from build123d import *

# Parameters (mm, degrees)
SKETCH1_R               = 0.5
SKETCH1_R_2             = 3.4
SKETCH1_R_3             = 2.2
SKETCH1_R_4             = 1.25
BASE_DEPTH              = 2.08
SKETCH1_3_R             = 3.4
SKETCH1_3_R_2           = 2.2
CONNECTION_DEPTH        = 2.5
CONNECTION_DEPTH_BACK   = 2.25
SKETCH2_W               = 9.1
SKETCH2_H               = 3.75
ALIGNMENT_CHANNEL_DEPTH = 10


with BuildPart() as part:
    # Sketch1 → Base (new body)
    with BuildSketch(Plane.XY):
        with BuildLine():
            ThreePointArc((16.424, -1.942221409), (18.2, 0), (16.424, 1.942221409))
            Line((16.424, 1.942221409), (0.303384615, 3.386437328))
            ThreePointArc((0.303384615, 3.386437328), (2.509134083, 2.294394507), (3.4, 0))
            ThreePointArc((3.4, 0), (2.509134083, -2.294394507), (0.303384615, -3.386437328))
            Line((0.303384615, -3.386437328), (16.424, -1.942221409))
        make_face()
        with Locations((5.1, 0)):
            Circle(SKETCH1_R, mode=Mode.SUBTRACT)
        with Locations((6.983333333, 0)):
            Circle(SKETCH1_R, mode=Mode.SUBTRACT)
        with Locations((8.866666667, 0)):
            Circle(SKETCH1_R, mode=Mode.SUBTRACT)
        with Locations((10.75, 0)):
            Circle(SKETCH1_R, mode=Mode.SUBTRACT)
        with Locations((12.633333333, 0)):
            Circle(SKETCH1_R, mode=Mode.SUBTRACT)
        with Locations((14.516666667, 0)):
            Circle(SKETCH1_R, mode=Mode.SUBTRACT)
        with Locations((16.4, 0)):
            Circle(SKETCH1_R, mode=Mode.SUBTRACT)
        Circle(SKETCH1_R_2)
        Circle(SKETCH1_R_3, mode=Mode.SUBTRACT)
        Circle(SKETCH1_R_3)
        Circle(SKETCH1_R_4, mode=Mode.SUBTRACT)
    extrude(amount=BASE_DEPTH)

    # Sketch1_3 → Connection (add, two sides)
    with BuildSketch(Plane.XY) as connection_sk:
        Circle(SKETCH1_3_R)
        Circle(SKETCH1_3_R_2, mode=Mode.SUBTRACT)
    extrude(amount=CONNECTION_DEPTH)
    extrude(connection_sk.sketch, amount=-CONNECTION_DEPTH_BACK)

    # Sketch2 → Alignment channel (cut)
    with BuildSketch(Plane(origin=(0, 0, 0), x_dir=(-1, 0, 0), z_dir=(0, 0, -1))):
        with Locations((-8.575, 0)):
            Rectangle(SKETCH2_W, SKETCH2_H)
    extrude(amount=-ALIGNMENT_CHANNEL_DEPTH, mode=Mode.SUBTRACT)


solid = part.part
Verification items for the finished model (mm, model axes). A direction names the side the tool comes from. Give positions to 0.01 mm unless a question says otherwise; leave off trailing zeros. Loops run counter-clockwise (first coordinate to the right, second up) from the corner with the lowest first, then second, coordinate; pieces in that order, holes last. Notation, with made-up numbers: (-25.75, 69) - (-10.75, 69) arc R13 cw to (-10.75, 80) - close; hole circle Ø6 at (56, -36). An arc over 180 degrees is marked (long way). Write item = value, one per line. Start each with the question number.
Q1. Cross-section at D-D, the plane x = 5.5. Enter the section's corners in (y, z) (3 decimals), and give its area (3 significant figures).
Q2. Thickness scan on line 1 (Y direction, x = 0, z = 0.6); line 2 (Y direction, x = 0, z = -1.45); line 3 (X direction, y = -0.75, z = 1.15) (3 decimals). Record the ranges inside material, lowest first.
Q3. Cross-section at A-A, the plane x = 0. Enter the section's corners in (y, z).
Q4. Cross-section at C-C, the plane y = -1. Enter the section's corners in (x, z) (3 decimals).
Q5. Depth check by flat-ended pin: P1, Ø2, axis at x = 8, z = 0, coming from the -Y side; P2, Ø0.5, axis at y = 1, z = 1, coming from the -X side; P3, Ø2, axis at x = 1, y = 0.5, coming from the -Z side. Enter the tip coordinate at first touch or a pass-through.
Q6. Tool access check on faces 1 (the face through (2.1, 0.66, -1.11)), 2 (the face through (18.2, 0, 1)), 3 (the face through (4.025, 0, 1)), 4 (the face through (2.1, 0.66, 2.29)), 5 (the face through (-2, 2, 2.5)). Record the directions out of +Z, -Z, +X, -X, +Y, -Y that give a thin tool (end or side, any length) a straight path to the whole face; none if there is none.
Q7. Cross-section at B-B, the plane z = 1.8. Enter the section's corners in (x, y) (3 decimals), and give its area (3 significant figures).
Q8. Mould release check, pull along X, two halves, no side actions. Record for faces 6 (the face through (-3.4, 0.1, 0.2)), 7 (the face through (9, 1.875, 1)), 8 (the face through (-2, 2, -2.25)), 9 (the face through (14.017, 0.022, 1.025)): released by +X, released by -X, zero draft, split by the parting line, or undercut.
Answer key:
q1.outline = (-2.921, 0) - (-1.875, 0) - (-1.875, 2.08) - (-2.921, 2.08) - close; (1.875, 0) - (2.921, 0) - (2.921, 2.08) - (1.875, 2.08) - close
q1.area = 4.35 mm^2
q2.line_1 = -3.4 to -1.25, 1.25 to 3.4
q2.line_2 = -3.4 to -2.2, 2.2 to 3.4
q2.line_3 = -3.316 to -1, 1 to 4.025, 13.125 to 18.05
q3.outline = (-3.4, -2.25) - (-2.2, -2.25) - (-2.2, 0) - (-1.25, 0) - (-1.25, 2.08) - (-2.2, 2.08) - (-2.2, 2.5) - (-3.4, 2.5) - close; (1.25, 0) - (2.2, 0) - (2.2, -2.25) - (3.4, -2.25) - (3.4, 2.5) - (2.2, 2.5) - (2.2, 2.08) - (1.25, 2.08) - close
q4.outline = (-3.25, -2.25) - (-1.96, -2.25) - (-1.96, 0) - (-0.75, 0) - (-0.75, 2.08) - (-1.96, 2.08) - (-1.96, 2.5) - (-3.25, 2.5) - close; (0.75, 0) - (1.96, 0) - (1.96, -2.25) - (3.25, -2.25) - (3.25, 0) - (4.025, 0) - (4.025, 2.08) - (3.25, 2.08) - (3.25, 2.5) - (1.96, 2.5) - (1.96, 2.08) - (0.75, 2.08) - close; (13.125, 0) - (17.924, 0) - (17.924, 2.08) - (13.125, 2.08) - close
q5.P1 = -2.79
q5.P2 = -3.32
q5.P3 = 0
q6.face_1 = -Z
q6.face_2 = +Z, -Z, +X
q6.face_3 = +Z, -Z
q6.face_4 = +Z
q6.face_5 = +Z, +X, -X, +Y, -Y
q7.outline = (0.303, -3.386) - (16.424, -1.942) arc R1.95 ccw to (16.424, 1.942) - (0.303, 3.386) arc R3.4 ccw (long way) to start; hole circle Ø2.5 at (0, 0); hole (4.025, -1.875) - (13.125, -1.875) - (13.125, -0.091) arc R0.5 ccw to (13.125, 0.091) - (13.125, 1.875) - (4.025, 1.875) - close; hole circle Ø1 at (14.517, 0); hole circle Ø1 at (16.4, 0)
q7.area = 70.8 mm^2
q8.face_6 = split by the parting line
q8.face_7 = undercut
q8.face_8 = zero draft
q8.face_9 = undercut
